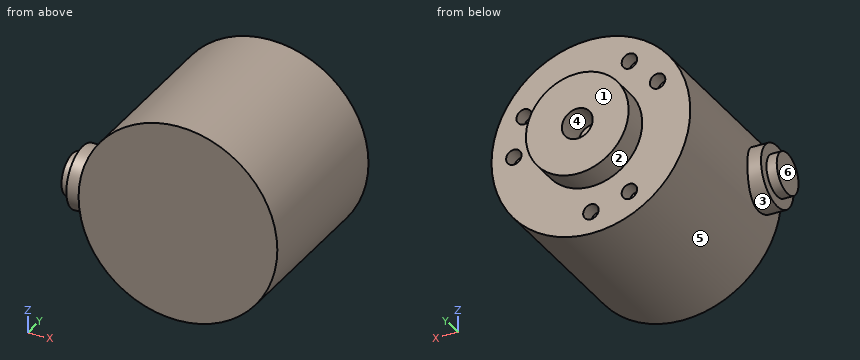
```python
from build123d import *

# Parameters (mm, degrees)
SKETCH2_R                = 19.35
BOSS_EXTRUDE1_DEPTH      = 33.5
SKETCH3_R                = 10
BOSS_EXTRUDE2_DEPTH      = 5
SKETCH4_R                = 1.5
CUT_EXTRUDE1_DEPTH       = 3
SKETCH5_R                = 3
CUT_EXTRUDE2_DEPTH       = 6
BOSS_EXTRUDE3_REACH      = 61.72
BOSS_EXTRUDE3_END_RADIUS = 19.35
SKETCH6_R                = 6
SKETCH7_R                = 4
BOSS_EXTRUDE4_DEPTH      = 2


with BuildPart() as part:
    # Sketch2 → Boss-Extrude1 (new body)
    with BuildSketch(Plane(origin=(0, 0, 0), x_dir=(1, 0, 0), z_dir=(0, 1, 0))):
        with Locations(Location((0, 0, 0), (0, 0, 270))):
            Circle(SKETCH2_R)
    extrude(amount=BOSS_EXTRUDE1_DEPTH)

    # Sketch3 → Boss-Extrude2 (add)
    with BuildSketch(Plane(origin=(0, 33.5, 0), x_dir=(1, 0, 0), z_dir=(0, 1, 0))):
        with Locations(Location((0, 0, 0), (0, 0, 270))):
            Circle(SKETCH3_R)
    extrude(amount=BOSS_EXTRUDE2_DEPTH)

    # Sketch4 → Cut-Extrude1 (cut)
    with BuildSketch(Plane(origin=(0, 33.5, 0), x_dir=(1, 0, 0), z_dir=(0, 1, 0))):
        with Locations(Location((15, 0, 0), (0, 0, 270))):
            Circle(SKETCH4_R)
        with Locations(Location((12.990381057, -7.5, 0), (0, 0, 270))):
            Circle(SKETCH4_R)
        with Locations(Location((0, 15, 0), (0, 0, 270))):
            Circle(SKETCH4_R)
        with Locations(Location((-12.990381057, -7.5, 0), (0, 0, 270))):
            Circle(SKETCH4_R)
        with Locations(Location((-7.5, -12.990381057, 0), (0, 0, 270))):
            Circle(SKETCH4_R)
        with Locations(Location((-7.5, 12.990381057, 0), (0, 0, 270))):
            Circle(SKETCH4_R)
    extrude(amount=-CUT_EXTRUDE1_DEPTH, mode=Mode.SUBTRACT)

    # Sketch5 → Cut-Extrude2 (cut)
    with BuildSketch(Plane(origin=(0, 38.5, 0), x_dir=(1, 0, 0), z_dir=(0, 1, 0))):
        with Locations(Location((0, 0, 0), (0, 0, 270))):
            Circle(SKETCH5_R)
    extrude(amount=-CUT_EXTRUDE2_DEPTH, mode=Mode.SUBTRACT)

    # Boss-Extrude3: up to this cylinder (the profile starts outside it)
    boss_extrude3_end = Plane(origin=(0, 6.5, 0), z_dir=(0, -1, 0)) * Cylinder(BOSS_EXTRUDE3_END_RADIUS, 163.14, mode=Mode.PRIVATE)
    # Sketch6 → Boss-Extrude3 (add, up to the surface)
    with BuildSketch(Plane(origin=(-22, 0, 0), x_dir=(0, 0, -1), z_dir=(1, 0, 0)), mode=Mode.PRIVATE) as boss_extrude3_sk1:
        with Locations(Location((0, 6.5, 0), (0, 0, 180))):
            Circle(SKETCH6_R)
    boss_extrude3_tool1 = extrude(boss_extrude3_sk1.sketch, amount=BOSS_EXTRUDE3_REACH, mode=Mode.PRIVATE) - boss_extrude3_end
    add(boss_extrude3_tool1.solids().sort_by_distance((-22, 6.5, 0))[0])

    # Sketch7 → Boss-Extrude4 (add)
    with BuildSketch(Plane.ZY.offset(22)):
        with Locations((0, 6.5)):
            Circle(SKETCH7_R)
    extrude(amount=BOSS_EXTRUDE4_DEPTH)


solid = part.part
```
Part model, mm, in its own coordinate system. Face numbers are marked on the shaded views. A direction names the side the tool comes from. Round coordinates to 2 decimals unless told otherwise and drop trailing zeros. Write each loop counter-clockwise with the first axis right and the second up, starting at its lowest first coordinate (ties: lowest second). Pieces come first, ordered by that corner, then holes.
Item 1: Cut at C-C, the plane x = -7.5. Give the cut face in (y, z).
Results:
outline: (0, -17.84) - (33.5, -17.84) - (33.5, -14.49) - (30.5, -14.49) - (30.5, -11.49) - (33.5, -11.49) - (33.5, -6.61) - (38.5, -6.61) - (38.5, 6.61) - (33.5, 6.61) - (33.5, 11.49) - (30.5, 11.49) - (30.5, 14.49) - (33.5, 14.49) - (33.5, 17.84) - (0, 17.84) - close
Item 2: Two-plate mould, pull along X, no slides. Class the marked faces 4, 5 and 6: +X half, -X half, draft (parallel to the pull), parting line (faces both ways), or undercut.
Results:
face 4: undercut
face 5: parting line
face 6: -X half
Item 3: Probe L1, parallel to Y at x = -10, z = 11; L2, parallel to X at y = 31.4, z = 0; L3, parallel to Y at x = 0, z = -14. List the from-to ranges inside material, lowest first.
Results:
L1: y = 0 to 33.5
L2: x = -19.35 to 13.5, 16.5 to 19.35
L3: y = 0 to 30.5
Item 4: Cut at D-D, the plane z = 0. Give the cut face in (x, y).
Results:
outline: (-24, 2.5) - (-22, 2.5) - (-22, 0.5) - (-19.35, 0.5) - (-19.35, 0) - (19.35, 0) - (19.35, 33.5) - (16.5, 33.5) - (16.5, 30.5) - (13.5, 30.5) - (13.5, 33.5) - (10, 33.5) - (10, 38.5) - (3, 38.5) - (3, 32.5) - (-3, 32.5) - (-3, 38.5) - (-10, 38.5) - (-10, 33.5) - (-19.35, 33.5) - (-19.35, 12.5) - (-22, 12.5) - (-22, 10.5) - (-24, 10.5) - close
Item 5: Which spindle directions (+Z, -Z, +X, -X, +Y, -Y) get a long thin tool onto all of the face, cutting with end or side? Do the marked faces 1, 2 and 3. Say none if no direction does.
Results:
face 1: +Z, -Z, +X, -X, +Y
face 2: +Y
face 3: -X
Item 6: Cut at B-B, the plane z = -5. Give the cut face in (x, y).
Results:
outline: (-22, 3.18) - (-18.69, 3.18) - (-18.69, 0) - (18.69, 0) - (18.69, 33.5) - (8.66, 33.5) - (8.66, 38.5) - (-8.66, 38.5) - (-8.66, 33.5) - (-18.69, 33.5) - (-18.69, 9.82) - (-22, 9.82) - close
Item 7: Cut at A-A, the plane y = 6.5. Give the cut face in (x, z), plus the area to 3 significant figures.
Results:
outline: (-24, -4) - (-22, -4) - (-22, -6) - (-18.4, -6) arc R19.35 ccw (long way) to (-18.4, 6) - (-22, 6) - (-22, 4) - (-24, 4) - close
area: 1,230 mm2
Item 8: Drop flat-ended pins along their axis: pin 1 Ø1.8 at (x, z) = (-7.5, 12.99) entering from +Y; pin 2 Ø5 at (x, z) = (12.99, 7.5) entering from +Y; pin 3 Ø1.5 at (x, y) = (-16.5, 4) entering from +Z. Give the stop position or say it passes through.
Results:
pin 1: stops at y = 30.5
pin 2: stops at y = 33.5
pin 3: stops at z = 11.24
